Geometry: final body of the model. Coordinates: model frame, mm. A direction names the side the tool comes from. Give positions to 0.01 mm unless a question says otherwise; leave off trailing zeros. Put each result on its own line as item: value. Start each with the question number.
1. Set-up query: faces 1 (the flat face through (-9, -10, 700)), 2 (the flat face through (-12.3, 0, 345)). Return all of +Z, -Z, +X, -X, +Y, -Y with unobstructed straight access to the full face (end or side cutting, diameter ignored); none if empty.
2. First-contact query: P1, Ø2, axis at x = 22, z = 617.5, coming from the +Y side; P2, Ø1.5, axis at y = -0.5, z = 606, coming from the -X side; P3, Ø0.8, axis at y = 17, z = 397, coming from the +X side. Flat tips, straight axial feed; report the tip coordinate or a pass-through.
3. Ray query, line 1 along Y through (x, z) = (33.5, 259); line 2 along X through (y, z) = (4.5, 140); line 3 along X through (y, z) = (-14, 271). Return the intervals inside material, ascending. Write a range as from..to.
4. Section A-A on z = 482. Count the separate pieces of the cut face and the enclosed holes in it, plus the area to 3 significant figures.
5. Mould query, pull axis Y, two halves, no side actions, for faces 3 (the flat face through (0, -20, 345)), 4 (the flat face through (-40, 10, 345)), 5 (the flat face through (-20, -7.7, 345)), 6 (the flat face through (0, 20, 345)). Classes: pulls with the +Y half, pulls with the -Y half, needs draft (parallel to the pull), parting line crosses it, or undercut.
from build123d import *

# Parameters (mm, degrees)
SKETCH1_R           = 3.4
BOSS_EXTRUDE1_DEPTH = 700


with BuildPart() as part:
    # Sketch1 → Boss-Extrude1 (new body)
    with BuildSketch(Plane.XY):
        with BuildLine():
            Line((24.1, -20), (35.5, -20))
            ThreePointArc((35.5, -20), (38.681980515, -18.681980515), (40, -15.5))
            Line((40, -15.5), (40, -4.1))
            Line((40, -4.1), (35.5, -4.1))
            Line((35.5, -4.1), (35.5, -6.6))
            Line((35.5, -6.6), (38, -6.6))
            Line((38, -6.6), (38, -10.25))
            Line((38, -10.25), (32.017766953, -10.25))
            Line((32.017766953, -10.25), (27.7, -5.932233047))
            Line((27.7, -5.932233047), (27.7, 5.932233047))
            Line((27.7, 5.932233047), (32.017766953, 10.25))
            Line((32.017766953, 10.25), (38, 10.25))
            Line((38, 10.25), (38, 6.6))
            Line((38, 6.6), (35.5, 6.6))
            Line((35.5, 6.6), (35.5, 4.1))
            Line((35.5, 4.1), (40, 4.1))
            Line((40, 4.1), (40, 15.5))
            ThreePointArc((40, 15.5), (38.681980515, 18.681980515), (35.5, 20))
            Line((35.5, 20), (24.1, 20))
            Line((24.1, 20), (24.1, 15.5))
            Line((24.1, 15.5), (26.6, 15.5))
            Line((26.6, 15.5), (26.6, 18))
            Line((26.6, 18), (30.25, 18))
            Line((30.25, 18), (30.25, 12.017766953))
            Line((30.25, 12.017766953), (25.932233047, 7.7))
            Line((25.932233047, 7.7), (14.067766953, 7.7))
            Line((14.067766953, 7.7), (9.75, 12.017766953))
            Line((9.75, 12.017766953), (9.75, 18))
            Line((9.75, 18), (13.4, 18))
            Line((13.4, 18), (13.4, 15.5))
            Line((13.4, 15.5), (15.9, 15.5))
            Line((15.9, 15.5), (15.9, 20))
            Line((15.9, 20), (-15.9, 20))
            Line((-15.9, 20), (-15.9, 15.5))
            Line((-15.9, 15.5), (-13.4, 15.5))
            Line((-13.4, 15.5), (-13.4, 18))
            Line((-13.4, 18), (-9.75, 18))
            Line((-9.75, 18), (-9.75, 12.017766953))
            Line((-9.75, 12.017766953), (-14.067766953, 7.7))
            Line((-14.067766953, 7.7), (-25.932233047, 7.7))
            Line((-25.932233047, 7.7), (-30.25, 12.017766953))
            Line((-30.25, 12.017766953), (-30.25, 18))
            Line((-30.25, 18), (-26.6, 18))
            Line((-26.6, 18), (-26.6, 15.5))
            Line((-26.6, 15.5), (-24.1, 15.5))
            Line((-24.1, 15.5), (-24.1, 20))
            Line((-24.1, 20), (-35.5, 20))
            ThreePointArc((-35.5, 20), (-38.681980515, 18.681980515), (-40, 15.5))
            Line((-40, 15.5), (-40, 4.1))
            Line((-40, 4.1), (-35.5, 4.1))
            Line((-35.5, 4.1), (-35.5, 6.6))
            Line((-35.5, 6.6), (-38, 6.6))
            Line((-38, 6.6), (-38, 10.25))
            Line((-38, 10.25), (-32.017766953, 10.25))
            Line((-32.017766953, 10.25), (-27.7, 5.932233047))
            Line((-27.7, 5.932233047), (-27.7, -5.932233047))
            Line((-27.7, -5.932233047), (-32.017766953, -10.25))
            Line((-32.017766953, -10.25), (-38, -10.25))
            Line((-38, -10.25), (-38, -6.6))
            Line((-38, -6.6), (-35.5, -6.6))
            Line((-35.5, -6.6), (-35.5, -4.1))
            Line((-35.5, -4.1), (-40, -4.1))
            Line((-40, -4.1), (-40, -15.5))
            ThreePointArc((-40, -15.5), (-38.681980515, -18.681980515), (-35.5, -20))
            Line((-35.5, -20), (-24.1, -20))
            Line((-24.1, -20), (-24.1, -15.5))
            Line((-24.1, -15.5), (-26.6, -15.5))
            Line((-26.6, -15.5), (-26.6, -18))
            Line((-26.6, -18), (-30.25, -18))
            Line((-30.25, -18), (-30.25, -12.017766953))
            Line((-30.25, -12.017766953), (-25.932233047, -7.7))
            Line((-25.932233047, -7.7), (-14.067766953, -7.7))
            Line((-14.067766953, -7.7), (-9.75, -12.017766953))
            Line((-9.75, -12.017766953), (-9.75, -18))
            Line((-9.75, -18), (-13.4, -18))
            Line((-13.4, -18), (-13.4, -15.5))
            Line((-13.4, -15.5), (-15.9, -15.5))
            Line((-15.9, -15.5), (-15.9, -20))
            Line((-15.9, -20), (15.9, -20))
            Line((15.9, -20), (15.9, -15.5))
            Line((15.9, -15.5), (13.4, -15.5))
            Line((13.4, -15.5), (13.4, -18))
            Line((13.4, -18), (9.75, -18))
            Line((9.75, -18), (9.75, -12.017766953))
            Line((9.75, -12.017766953), (14.067766953, -7.7))
            Line((14.067766953, -7.7), (25.932233047, -7.7))
            Line((25.932233047, -7.7), (30.25, -12.017766953))
            Line((30.25, -12.017766953), (30.25, -18))
            Line((30.25, -18), (26.6, -18))
            Line((26.6, -18), (26.6, -15.5))
            Line((26.6, -15.5), (24.1, -15.5))
            Line((24.1, -15.5), (24.1, -20))
        make_face()
        with Locations((-20, 0)):
            Circle(SKETCH1_R, mode=Mode.SUBTRACT)
        with Locations((20, 0)):
            Circle(SKETCH1_R, mode=Mode.SUBTRACT)
        with BuildLine():
            Line((38, -15.5), (38, -11.75))
            Line((38, -11.75), (31.75, -11.75))
            Line((31.75, -11.75), (31.75, -18))
            Line((31.75, -18), (35.5, -18))
            ThreePointArc((35.5, -18), (37.267766953, -17.267766953), (38, -15.5))
        make_face(mode=Mode.SUBTRACT)
        with BuildLine():
            Line((-38, 15.5), (-38, 11.75))
            Line((-38, 11.75), (-31.75, 11.75))
            Line((-31.75, 11.75), (-31.75, 18))
            Line((-31.75, 18), (-35.5, 18))
            ThreePointArc((-35.5, 18), (-37.267766953, 17.267766953), (-38, 15.5))
        make_face(mode=Mode.SUBTRACT)
        Polygon((-7.25, -10.982233047), (-7.25, -17.8), (7.25, -17.8), (7.25, -10.982233047), (12.3, -5.932233047), (12.3, 5.932233047), (7.25, 10.982233047), (7.25, 17.8), (-7.25, 17.8), (-7.25, 10.982233047), (-12.3, 5.932233047), (-12.3, -5.932233047), align=None, mode=Mode.SUBTRACT)
        with BuildLine():
            Line((-35.5, -18), (-31.75, -18))
            Line((-31.75, -18), (-31.75, -11.75))
            Line((-31.75, -11.75), (-38, -11.75))
            Line((-38, -11.75), (-38, -15.5))
            ThreePointArc((-38, -15.5), (-37.267766953, -17.267766953), (-35.5, -18))
        make_face(mode=Mode.SUBTRACT)
        with BuildLine():
            Line((35.5, 18), (31.75, 18))
            Line((31.75, 18), (31.75, 11.75))
            Line((31.75, 11.75), (38, 11.75))
            Line((38, 11.75), (38, 15.5))
            ThreePointArc((38, 15.5), (37.267766953, 17.267766953), (35.5, 18))
        make_face(mode=Mode.SUBTRACT)
    extrude(amount=BOSS_EXTRUDE1_DEPTH)


solid = part.part
Resolved:
1. face 1: +Z, +X, -X, +Y, -Y
1. face 2: +Z, -Z
2. P1: y = 7.7
2. P2: x = -27.7
2. P3: x = 39.86
3. line 1: -20..-18, -11.75..-10.25, 10.25..11.75, 18..20
3. line 2: -40..-35.5, -27.7..-12.3, 12.3..27.7, 35.5..40
3. line 3: -40..-38, -31.75..-30.25, -9.75..-7.25, 7.25..9.75, 30.25..31.75, 38..40
4. separate pieces: 1
4. enclosed holes: 7
4. area: 1,090 mm^2
5. face 3: pulls with the -Y half
5. face 4: needs draft
5. face 5: undercut
5. face 6: pulls with the +Y half
